```python
from build123d import *

# Parameters (mm, degrees)
F0_R     = 12.7
F1_DEPTH = 6.35


with BuildPart() as f1:
    # F0 (on Front) → F1 (new body)
    with BuildSketch(Plane.XZ):
        with BuildLine():
            ThreePointArc((-75.109355, -31.75024), (-59.33875, -34.579478), (-46.125851, -43.642363))
            ThreePointArc((-46.125851, -43.642363), (0.007907, -63.5), (46.136719, -43.630874))
            ThreePointArc((46.136719, -43.630874), (59.347524, -34.564632), (75.117614, -31.731545))
            ThreePointArc((75.117614, -31.731545), (107.95, 0), (75.117614, 31.731545))
            ThreePointArc((75.117614, 31.731545), (59.347524, 34.564632), (46.136719, 43.630874))
            ThreePointArc((46.136719, 43.630874), (0.007907, 63.5), (-46.125851, 43.642363))
            ThreePointArc((-46.125851, 43.642363), (-59.33875, 34.579478), (-75.109355, 31.75024))
            ThreePointArc((-75.109355, 31.75024), (-107.968966, 0), (-75.109355, -31.75024))
        make_face()
        with Locations((-76.2, 0)):
            Circle(F0_R, mode=Mode.SUBTRACT)
        with BuildLine():
            ThreePointArc((-44.442095, 0.838267), (0.419152, 44.448024), (44.45, 0))
            ThreePointArc((44.45, 0), (0.419152, -44.448024), (-44.442095, -0.838267))
            ThreePointArc((-44.442095, -0.838267), (-44.45, 0), (-44.442095, 0.838267))
        make_face(mode=Mode.SUBTRACT)
        with Locations((76.2, 0)):
            Circle(F0_R, mode=Mode.SUBTRACT)
    extrude(amount=F1_DEPTH)


solid = f1.part
```
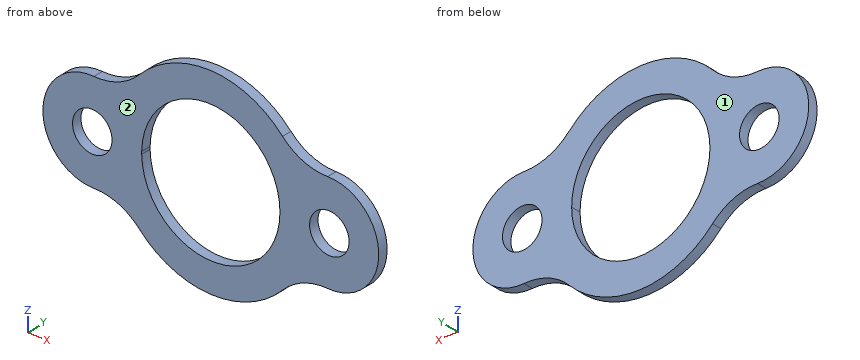
The model under review builds one solid part; all positions refer to its coordinate system, in mm. Face numbers are marked on the shaded views. Round coordinates to 2 decimals unless told otherwise and drop trailing zeros. Loops run counter-clockwise (first coordinate to the right, second up) from the corner with the lowest first, then second, coordinate; pieces in that order, holes last. Notation, with made-up numbers: M 56,54 L 104,54 A12 ccw 104,66 Z; hole C 35.25,34 d4. An arc over 180 degrees is marked long. Answer as a JSON object with one key per item and string values.
(1) Take a section at C-C on y = -5.25. Give the boundary of the cut face in (x, z).
Resolved:
{"outline": "M -75.11,-31.75 A38.1 cw -46.13,-43.64 A63.5 ccw 46.14,-43.63 A38.1 cw 75.12,-31.73 A31.75 ccw long 75.12,31.73 A38.1 cw 46.14,43.63 A63.5 ccw -46.13,43.64 A38.1 cw -75.11,31.75 A31.77 ccw long Z; hole C -76.2,0 d25.4; hole M -44.44,-0.84 A44.45 ccw long -44.44,0.84 A44.45 ccw Z; hole C 76.2,0 d25.4"}
(2) To check wall thickness, follow line 1 along Z through (x, y) = (76.2, -4.5); line 2 along Z through (x, y) = (-76.2, -1.75); line 3 along X through (y, z) = (-3, -14.5). State the ranges of each line that lie inside material, in increasing order.
Resolved:
{"line 1": "-31.75 to -12.7, 12.7 to 31.75", "line 2": "-31.77 to -12.7, 12.7 to 31.77", "line 3": "-104.47 to -42.02, 42.02 to 104.45"}
(3) Draft analysis for pull direction Y (two halves, no side actions). For the marked faces 1 and 2, state which applies: released by +Y, released by -Y, zero draft, split by the parting line, or undercut.
Resolved:
{"face 1": "released by +Y", "face 2": "released by -Y"}
(4) Take a section at D-D on z = 48. Give the boundary of the cut face in (x, y).
Resolved:
{"outline": "M -41.57,-6.35 L 41.57,-6.35 L 41.57,0 L -41.57,0 Z"}
(5) Clearance check with flat-ended pins moving along their axes: P1, Ø10, axis at x = -29, z = -24.5, coming from the -Y side; P2, Ø1, axis at y = -1.5, z = -38.5, coming from the -X side; P3, Ø1.5, axis at x = 60.5, y = -2.5, coming from the -Z side; P4, Ø3, axis at x = 33.5, y = -2, coming from the -Z side. State where each tip first meets the part, or that it passes through.
Resolved:
{"P1": "through", "P2": "x = -52.86", "P3": "z = -34.4", "P4": "z = -54.85"}
(6) Take a section at A-A on x = 0. Give the boundary of the cut face in (y, z).
Resolved:
{"outline": "M -6.35,-63.5 L 0,-63.5 L 0,-44.45 L -6.35,-44.45 Z; M -6.35,44.45 L 0,44.45 L 0,63.5 L -6.35,63.5 Z"}
(7) Take a section at B-B on z = -22. Give the boundary of the cut face in (x, y).
Resolved:
{"outline": "M -99.12,-6.35 L -38.62,-6.35 L -38.62,0 L -99.12,0 Z; M 38.62,-6.35 L 99.09,-6.35 L 99.09,0 L 38.62,0 Z"}
